```python
from build123d import *

# Parameters (mm, degrees)
SWEEP_THIN2_PROFILE_R   = 3.5
SWEEP_THIN2_PROFILE_R_2 = 2.5
SKETCH57_R              = 3.5
SKETCH57_R_2            = 3
BOSS_EXTRUDE1_DEPTH     = 17.5
CUT_EXTRUDE1_START      = -2
SKETCH59_R              = 3.5
CUT_EXTRUDE1_DEPTH      = 2


with BuildPart() as part:
    # Sweep-Thin2: sweep along a path in Sketch28
    with BuildLine(Plane.XY) as sweep_thin2_path:
        Line((-67, -51), (-67, -13))
        ThreePointArc((-67, -13), (-63.192388155, -3.807611845), (-54, 0))
        Line((-54, 0), (54, 0))
        ThreePointArc((54, 0), (63.192388155, -3.807611845), (67, -13))
        Line((67, -13), (67, -51))
    # Sweep-Thin2 profile (on start of the path) → Sweep-Thin2 (sweep)
    with BuildSketch(Plane(origin=(-67, -51, 0), x_dir=(1, 0, 0), z_dir=(0, 1, 0))):
        Circle(SWEEP_THIN2_PROFILE_R)
        Circle(SWEEP_THIN2_PROFILE_R_2, mode=Mode.SUBTRACT)
    sweep(path=sweep_thin2_path.line)

    # Sketch57 → Boss-Extrude1 (add)
    with BuildSketch(Plane.XY):
        with Locations(Location((0, 0, 0), (0, 0, 270))):
            Circle(SKETCH57_R)
        with Locations(Location((0, 0, 0), (0, 0, 180))):
            Circle(SKETCH57_R_2, mode=Mode.SUBTRACT)
    extrude(amount=BOSS_EXTRUDE1_DEPTH)

    # Sketch59 → Cut-Extrude1 (cut)
    with BuildSketch(Plane.XY.offset(CUT_EXTRUDE1_START)):
        with Locations(Location((0, 0, 0), (0, 0, 270))):
            Circle(SKETCH59_R)
    extrude(amount=CUT_EXTRUDE1_DEPTH, mode=Mode.SUBTRACT)


solid = part.part
```
CAD build for the part. Positions are in the model's coordinates, mm. A direction names the side the tool comes from. Give positions to 0.01 mm unless a question says otherwise; leave off trailing zeros. Loops run counter-clockwise (first coordinate to the right, second up) from the corner with the lowest first, then second, coordinate; pieces in that order, holes last. Notation, with made-up numbers: M -40,18 L -34,18 A37 ccw -34,54 Z; hole C -21.5,26 d7. An arc over 180 degrees is marked long. Use one line per item in the form item = value.
Item 1: Slice it at C-C (z = 8.5). List the corners of the cut face in (x, y).
Determined:
outline = C 0,0 d7; hole C 0,0 d6
Item 2: Slice it at A-A (y = -31). List the corners of the cut face in (x, z), plus the area to 3 significant figures.
Determined:
outline = C -67,0 d7; C 67,0 d7; hole C -67,0 d5; hole C 67,0 d5
area = 37.7 mm2
Item 3: Which spindle directions (+Z, -Z, +X, -X, +Y, -Y) get a long thin tool onto all of the face, cutting with end or side? Do faces 4 (the face through (-2.86, -0.9, 9.54)), 5 (the face through (-64.615, -31.734, -0.751)), 6 (the face through (0.76, -1.34, -2.11)), 7 (the face through (65, -51, -2)). Say none if no direction does.
Determined:
face_4 = +Z
face_5 = -Y
face_6 = none
face_7 = +Z, -Z, +X, -X, -Y
Item 4: Flat gauge pins, fed straight in: pin 1 (6 mm diameter, centred on y = 0, z = 0, fed in from -X); pin 2 (6 mm diameter, centred on x = -67, z = 0, fed in from +Y); pin 3 (0.7 mm diameter, centred on x = 0, y = 2.5, fed in from +Z). Where does each tip first touch, or does it go through?
Determined:
pin_1 = -67.12
pin_2 = 0.12
pin_3 = 2.76
Item 5: Two-plate mould, pull along Z, no slides. Class faces 1 (the face through (-3.5, 0, 1)), 2 (the face through (1, -3, 17.5)), 3 (the face through (-69, -51, 2)): pulls with the +Z half, pulls with the -Z half, needs draft (parallel to the pull), parting line crosses it, or undercut.
Determined:
face_1 = undercut
face_2 = pulls with the +Z half
face_3 = needs draft
Item 6: Drill centre lines: probe 1 along Y at (x, z) = (-15.5, 0); probe 2 along X at (y, z) = (-10, 2). Where is each one in solid material? Low to high. Write a range as from..to.
Determined:
probe_1 = -3.5..-2.5, 2.5..3.5
probe_2 = -69.59..-68.19, -65.1..-63.67, 63.67..65.1, 68.19..69.59
Item 7: Slice it at B-B (x = 47.5). List the corners of the cut face in (y, z), plus the area to 3 significant figures.
Determined:
outline = C 0,0 d7; hole C 0,0 d5
area = 18.8 mm2
